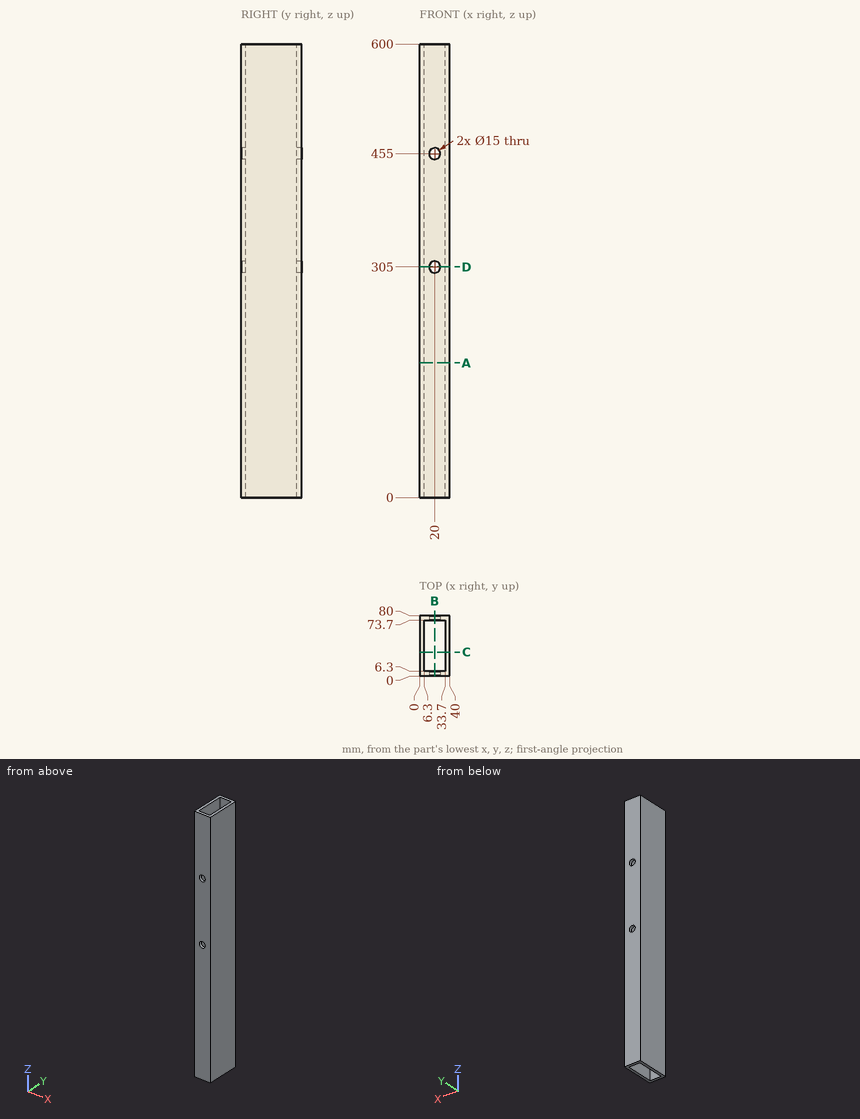
Print and shaded views of the part. All mm, measured from the part's lowest x, y and z. Give positions to 0.01 mm unless a question says otherwise; leave off trailing zeros. Order: outer loops, then holes, each group sorted by start corner. A loop starts at its lowest first (then second) coordinate and runs counter-clockwise, first axis right, second up. Notation, with made-up numbers: (-31, 60.5) - (-21, 60.5) arc R18 cw to (-21, 78.5) - close; hole circle Ø9 at (-35.75, 7.25). An arc over 180 degrees is marked (long way). One line per item, written item: value.
Item 1: Wall check: line 1 (Z direction, x = 20, y = 78.25); line 2 (Y direction, x = 19.5, z = 389.5); line 3 (X direction, y = 64.5, z = 558.5). Give the ranges that are in metal, low to high.
Response values:
line 1: 0 to 297.5, 312.5 to 447.5, 462.5 to 600
line 2: 0 to 6.3, 73.7 to 80
line 3: 0 to 6.3, 33.7 to 40
Item 2: Slice it at D-D (z = 305). List the corners of the cut face in (x, y).
Response values:
outline: (0, 0) - (12.5, 0) - (12.5, 6.3) - (6.3, 6.3) - (6.3, 73.7) - (12.5, 73.7) - (12.5, 80) - (0, 80) - close; (27.5, 0) - (40, 0) - (40, 80) - (27.5, 80) - (27.5, 73.7) - (33.7, 73.7) - (33.7, 6.3) - (27.5, 6.3) - close
Item 3: Slice it at C-C (y = 31.5). List the corners of the cut face in (x, z).
Response values:
outline: (0, 0) - (6.3, 0) - (6.3, 600) - (0, 600) - close; (33.7, 0) - (40, 0) - (40, 600) - (33.7, 600) - close
Item 4: Pin check, flat tips, straight feed: pin 1 Ø9 at (x, z) = (20, 305) entering from +Y; pin 2 Ø24 at (x, z) = (20, 305) entering from -Y. Stop position of each tip, or through.
Response values:
pin 1: through
pin 2: y = 0
Item 5: Slice it at A-A (z = 178). List the corners of the cut face in (x, y).
Response values:
outline: (0, 0) - (40, 0) - (40, 80) - (0, 80) - close; hole (6.3, 6.3) - (33.7, 6.3) - (33.7, 73.7) - (6.3, 73.7) - close
Item 6: Slice it at B-B (x = 20). List the corners of the cut face in (y, z).
Response values:
outline: (0, 0) - (6.3, 0) - (6.3, 297.5) - (0, 297.5) - close; (0, 312.5) - (6.3, 312.5) - (6.3, 447.5) - (0, 447.5) - close; (0, 462.5) - (6.3, 462.5) - (6.3, 600) - (0, 600) - close; (73.7, 0) - (80, 0) - (80, 297.5) - (73.7, 297.5) - close; (73.7, 312.5) - (80, 312.5) - (80, 447.5) - (73.7, 447.5) - close; (73.7, 462.5) - (80, 462.5) - (80, 600) - (73.7, 600) - close
